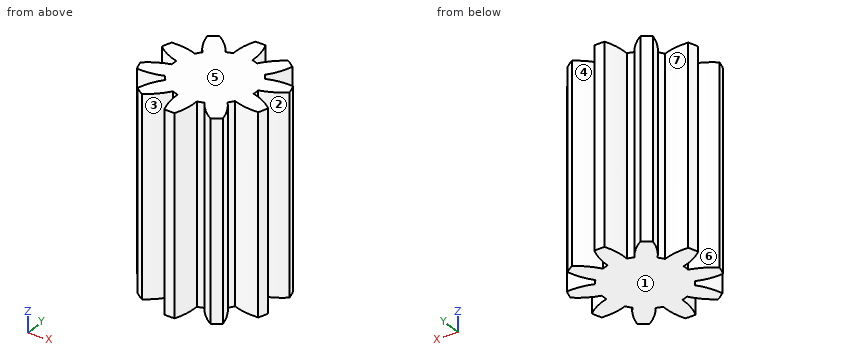
Autodesk Inventor part; units mm, degrees
ref_plane "Work Plane2" through (0, 0, 9) normal (0, 0, 1) x (1, 0, 0)
ref_plane "Work Plane8" through (0, 0, 0) normal (0.9510565, 0.309017, 0) x (0, 0, 1)
ref_plane "Work Plane9" through (0, 0, 0) normal (1, 0, 0) x (0, 1, 0)
sketch "Sketch1" plane through (0, 0, 0) normal (0, 0, 1) x (1, 0, 0)
  circle A0 centre (0, 0) radius 6
  dimension "d0" = 12
extrude "Extrusion1" add sketch "Sketch1" along normal blind 18
ref_plane "Work Plane2" through (0, 0, 9) normal (0, 0, 1) x (1, 0, 0)
sketch "Sketch2" plane through (0, 0, 0) normal (0, 0, -1) x (-1, 0, 0)
  circle A0 centre (0, 0) radius 6
  circle A1 centre (0, 0) radius 5
  dimension "d3" = 10
surface extrude "Pitch Diameter" sketch "Sketch2" against normal through all shown yes curves A1
ref_plane "Work Plane8" through (0, 0, 0) normal (0.9510565, 0.309017, 0) x (0, 0, 1)
ref_plane "Work Plane9" through (0, 0, 0) normal (1, 0, 0) x (0, 1, 0)
spur gear teeth "Spur Gear" teeth 10 pitch diameter 10 tip diameter 12 root diameter 7.5 face width 18 start plane through (0, 0, 0) normal (0, 0, -1) x (-1, 0, 0)
equation "\"d0\" = da_da"
equation "\"d1\" = da_b"
equation "\"d3\" = da_d"
equation "\"d16\" = da_aw"
equation "\"d43\" = da_aw"
equation "\"d46\" = da_aw"
properties part number "rs390_gear" material "Steel"
Geometry: final body of the model. Coordinates: model frame, mm. Face numbers are marked on the shaded views. A direction names the side the tool comes from. Give positions to 0.01 mm unless a question says otherwise; leave off trailing zeros. Write each loop counter-clockwise with the first axis right and the second up, starting at its lowest first coordinate (ties: lowest second). Pieces come first, ordered by that corner, then holes. Notation, with made-up numbers: M 17.5,-14.5 L 59.5,-14.5 A11 cw 59.5,0.5 Z; hole C 14.25,24 d2. An arc over 180 degrees is marked long. Answer in a Markdown table with one row per item. Add a question column.
(1) Reachability of the marked faces 4, 5, 6 and 7 from +Z, -Z, +X, -X, +Y, -Y: full face, straight path, thin tool, end or side. Return the list, or none.
(2) Section B-B on y = 1. Return loops of the section in (x, z).
(3) Ray query, line 1 (X direction, y = -4, z = 9.5); line 2 (X direction, y = 4.5, z = 14.5); line 3 (Y direction, x = -0.25, z = 6). Return the intervals inside material, ascending.
(4) Section C-C on x = -2. Return loops of the section in (y, z), and give its area (3 significant figures).
(5) First-contact query: pin 1 (1 mm diameter, centred on x = -2.5, z = 15.5, fed in from -Y); pin 2 (1.5 mm diameter, centred on y = -0.5, z = 9, fed in from -X); pin 3 (1 mm diameter, centred on x = -4, z = 15, fed in from +Y). Flat tips, straight axial feed; report the tip coordinate or a pass-through.
(6) Mould query, pull axis Y, two halves, no side actions, for the marked faces 1, 2 and 3. Classes: +Y half, -Y half, draft (parallel to the pull), parting line (faces both ways), or undercut.
(7) Section A-A on x = 3.5. Return loops of the section in (y, z).
Result set:
| question | item | result |
|---|---|---|
| 1 | face 4 | +Z, -Z, +Y |
| 1 | face 5 | +Z, +X, -X, +Y, -Y |
| 1 | face 6 | +Z, -Z, -X |
| 1 | face 7 | +Z, -Z |
| 2 | outline | M -5.3,0 L 5.3,0 L 5.3,18 L -5.3,18 Z |
| 3 | line 1 | x = -3.73 to -1.84, -0.88 to 0.88, 1.84 to 3.73 |
| 3 | line 2 | x = -3.88 to -2.32, -0.85 to 0.85, 2.32 to 3.88 |
| 3 | line 3 | y = -5.99 to 5.99 |
| 4 | outline | M -4.18,0 L 4.18,0 L 4.18,18 L -4.18,18 Z |
| 4 | area | 151 mm^2 |
| 5 | pin 1 | stops at y = -5.03 |
| 5 | pin 2 | stops at x = -5.65 |
| 5 | pin 3 | stops at y = 4.87 |
| 6 | face 1 | draft |
| 6 | face 2 | undercut |
| 6 | face 3 | -Y half |
| 7 | outline | M -4.87,0 L -3.46,0 L -3.46,18 L -4.87,18 Z; M -2.06,0 L 2.06,0 L 2.06,18 L -2.06,18 Z; M 3.46,0 L 4.87,0 L 4.87,18 L 3.46,18 Z |
